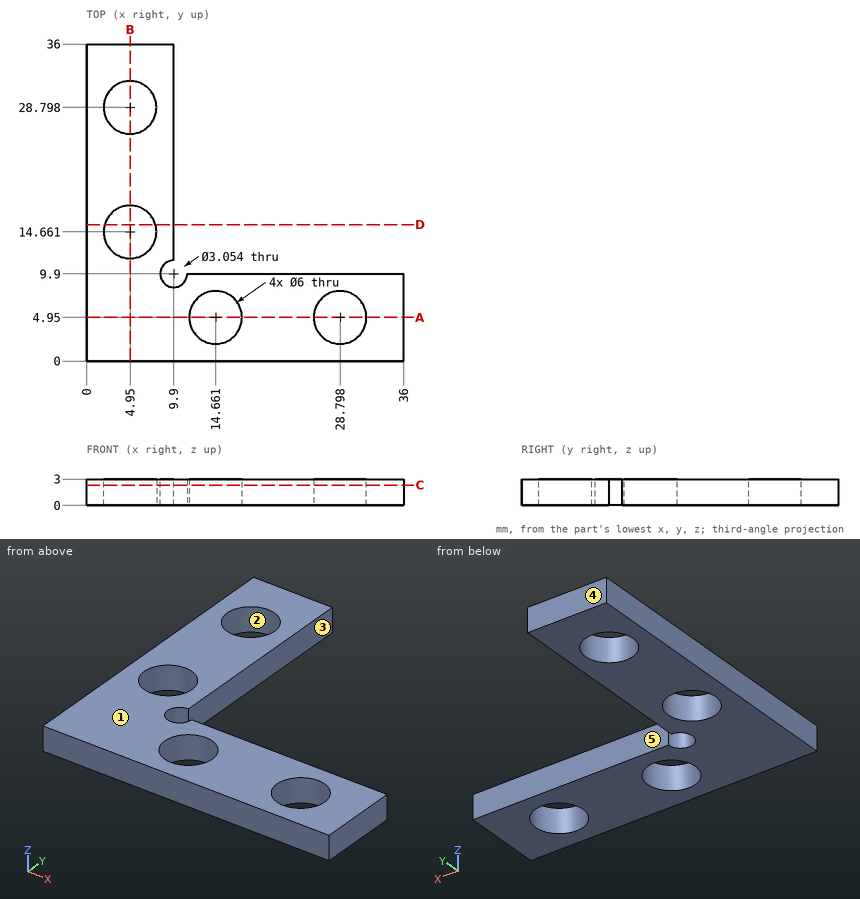
Source: three-view drawing plus pictorial views. Frame: mm from the lowest corner of the part. A direction names the side the tool comes from. Round coordinates to 2 decimals unless told otherwise and drop trailing zeros. Loops run counter-clockwise (first coordinate to the right, second up) from the corner with the lowest first, then second, coordinate; pieces in that order, holes last. Notation, with made-up numbers: M 49,18 L 99,18 A18 ccw 99,46 Z; hole C -6.5,-31 d2. An arc over 180 degrees is marked long. Answer as CSV lines item,"result". Start each with the question number.
(1) Line query: line 1 (X direction, y = 4.95, z = 1.7); line 2 (Y direction, x = 5.5, z = 2.8). Output: solid intervals per line, ascending. Write a range as [from, to].
(2) Section A-A, the plane y = 4.95. Output: boundary loops of the cut face in (x, z).
(3) Reachability of the marked faces 4 and 5 from +Z, -Z, +X, -X, +Y, -Y: full face, straight path, thin tool, end or side. Return the list, or none.
(4) Section C-C, the plane z = 2.3. State how many separate pieces and enclosed holes the cut face has, plus the area to 3 significant figures.
(5) Section D-D, the plane y = 15.5. Output: boundary loops of the cut face in (x, z).
(6) Draft query along X for the marked faces 1, 2 and 3. Return one class per face: released by +X, released by -X, zero draft, split by the parting line, or undercut.
(7) First-contact query: pin 1 (1.5 mm diameter, centred on y = 10, z = 1.5, fed in from -X). Flat tip, straight axial feed; report the tip coordinate or a pass-through.
Values found:
1,line 1,"x = [0, 11.66], [17.66, 25.8], [31.8, 36]"
1,line 2,"y = [0, 11.71], [17.61, 25.85], [31.75, 36]"
2,outline,"M 0,0 L 11.66,0 L 11.66,3 L 0,3 Z; M 17.66,0 L 25.8,0 L 25.8,3 L 17.66,3 Z; M 31.8,0 L 36,0 L 36,3 L 31.8,3 Z"
3,face 4,"+Z, -Z, +X, -X, +Y"
3,face 5,"+Z, -Z, +X, +Y"
4,separate pieces,"1"
4,enclosed holes,"4"
4,area,"496 mm²"
5,outline,"M 0,0 L 2.07,0 L 2.07,3 L 0,3 Z; M 7.83,0 L 9.9,0 L 9.9,3 L 7.83,3 Z"
6,face 1,"zero draft"
6,face 2,"undercut"
6,face 3,"released by +X"
7,pin 1,"stops at x = 0"
